from build123d import *

# Parameters (mm, degrees)
F0_W     = 56.6928
F0_H     = 45.7454
F1_DEPTH = 7.9756
F3_D     = 2.3876
F4_W     = 24.8666
F4_H     = 24.8666
F5_DEPTH = 4.9784


with BuildPart() as f1:
    # F0 (on Front) → F1 (new body)
    with BuildSketch(Plane.XZ):
        with Locations((-17.6647957414, 3.0100650459)):
            Rectangle(F0_W, F0_H)
    extrude(amount=F1_DEPTH)

    # F3 (through all)
    with Locations(Plane.XZ.offset(7.9756)):
        with Locations((-43.5219957414, 20.9043650459), (8.1924042586, 20.9043650459), (8.1924042586, -14.8842349541), (-43.5219957414, -14.8842349541)):
            Hole(F3_D / 2)

    # F4 (on face) → F5 (cut)
    with BuildSketch(Plane.XZ.offset(7.9756)):
        with Locations((-27.5072957414, 3.0100650459)):
            Rectangle(F4_W, F4_H)
    extrude(amount=-F5_DEPTH, mode=Mode.SUBTRACT)


solid = f1.part
Input: part model. Units: mm. Frame: model coordinates. A direction names the side the tool comes from. Round coordinates to 2 decimals unless told otherwise and drop trailing zeros. Write each loop counter-clockwise with the first axis right and the second up, starting at its lowest first coordinate (ties: lowest second). Pieces come first, ordered by that corner, then holes.
1) Cut plane B-B (y = -6). Return the cut outline in (x, z).
2) Reachability of faces 5 (the flat face through (-28, -6, -9.423)), 6 (the flat face through (-18, -4, -19.863)) from +Z, -Z, +X, -X, +Y, -Y: full face, straight path, thin tool, end or side. Return the list, or none.
3) Draft query along X for faces 1 (the flat face through (-28, -6, 15.443)), 2 (the flat face through (-12, -7.976, 3)), 3 (the cylindrical face through (-44.66, -3.93, -14.53)), 4 (the flat face through (-46.011, -4, 3)). Return one class per face: pulls with the +X half, pulls with the -X half, needs draft (parallel to the pull), parting line crosses it, or undercut.
4) Cut plane C-C (x = -24.5). Return the cut outline in (y, z), then the cut area to 3 significant figures.
5) Contact query for flat-ended pins moving along their axis: P1, Ø4, axis at x = -43.52, z = 20.9, coming from the -Y side; P2, Ø2, axis at x = -19.5, z = -2, coming from the -Y side. Output: stop coordinate, or through.
6) Ray query, L1, parallel to X at y = -2.75, z = -15; L2, parallel to Z at x = -36.5, y = -5.5; L3, parallel to X at y = -6.5, z = 10. Return the intervals inside material, ascending.
7) Cut plane A-A (z = 8). Return the cut outline in (x, y).
Geometry says:
1. outline: (-46.01, -19.86) - (10.68, -19.86) - (10.68, 25.88) - (-46.01, 25.88) - close; hole circle Ø2.39 at (-43.52, -14.88); hole circle Ø2.39 at (-43.52, 20.9); hole (-39.94, -9.42) - (-15.07, -9.42) - (-15.07, 15.44) - (-39.94, 15.44) - close; hole circle Ø2.39 at (8.19, -14.88); hole circle Ø2.39 at (8.19, 20.9)
2. face 5: -Y
2. face 6: -Z, +X, -X, +Y, -Y
3. face 1: undercut
3. face 2: needs draft
3. face 3: undercut
3. face 4: pulls with the -X half
4. outline: (-7.98, -19.86) - (0, -19.86) - (0, 25.88) - (-7.98, 25.88) - (-7.98, 15.44) - (-3, 15.44) - (-3, -9.42) - (-7.98, -9.42) - close
4. area: 241 mm2
5. P1: stops at y = -7.98
5. P2: stops at y = -3
6. L1: x = -46.01 to -44.71, -42.33 to 7, 9.38 to 10.68
6. L2: z = -19.86 to -9.42, 15.44 to 25.88
6. L3: x = -46.01 to -39.94, -15.07 to 10.68
7. outline: (-46.01, -7.98) - (-39.94, -7.98) - (-39.94, -3) - (-15.07, -3) - (-15.07, -7.98) - (10.68, -7.98) - (10.68, 0) - (-46.01, 0) - close
